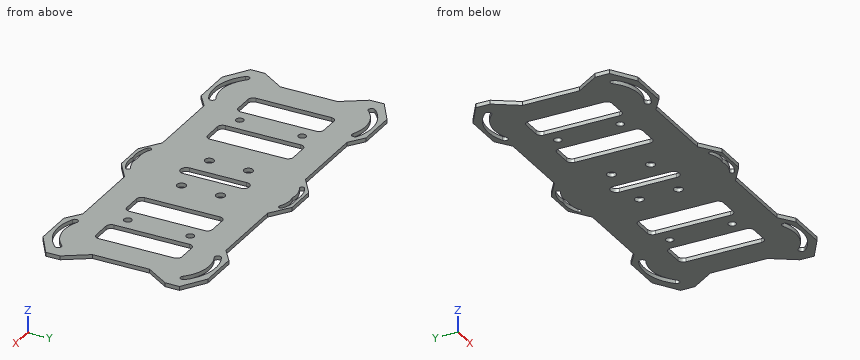
```python
from build123d import *

# Parameters (mm, degrees)
SCHIZZO1_R                   = 1.5
ESTRUSIONE_ESTRUSIONE1_DEPTH = 0.75
SKETCH1_R                    = 1.75
CUT_EXTRUDE1_DEPTH           = 1
CUT_EXTRUDE1_DEPTH_BACK      = 2.5


with BuildPart() as part:
    # Schizzo1 → Estrusione-Estrusione1 (new body, symmetric)
    with BuildSketch(Plane.XY):
        Polygon((-43.5, -27.5), (-13.615232638, -27.5), (-5.964504028, -32.859521299), (5.964504028, -32.859521299), (13.615232638, -27.5), (43.5, -27.5), (49.293787181, -31.722358535), (64.293787181, -31.722358535), (73.508072858, -25.714285677), (73.508072858, -20.214285677), (67.5, -11), (67.5, 11), (73.508072858, 20.214285677), (73.508072858, 25.714285677), (64.293787181, 31.722358535), (49.293787181, 31.722358535), (43.5, 27.5), (13.615232638, 27.5), (5.964504028, 32.859521299), (-5.964504028, 32.859521299), (-13.615232638, 27.5), (-43.5, 27.5), (-49.293787181, 31.722358535), (-64.293787181, 31.722358535), (-73.508072858, 25.714285677), (-73.508072858, 20.214285677), (-67.5, 11), (-67.5, -11), (-73.508072858, -20.214285677), (-73.508072858, -25.714285677), (-64.293787181, -31.722358535), (-49.293787181, -31.722358535), align=None)
        with BuildLine():
            ThreePointArc((-48.754479002, -28.623738791), (-59.172775767, -30.009764998), (-68.405644393, -24.988200197))
            ThreePointArc((-68.405644393, -24.988200197), (-68.356417198, -23.226138607), (-66.594355607, -23.275365801))
            ThreePointArc((-66.594355607, -23.275365801), (-58.719274878, -27.558458065), (-49.83309536, -26.376261209))
            ThreePointArc((-49.83309536, -26.376261209), (-48.17004839, -26.960691821), (-48.754479002, -28.623738791))
        make_face(mode=Mode.SUBTRACT)
        with Locations((-40.191447808, -12)):
            Circle(SCHIZZO1_R, mode=Mode.SUBTRACT)
        with BuildLine():
            ThreePointArc((0, -31.496185519), (-4.133745369, -31.563971562), (-8.018095478, -30.148249145))
            ThreePointArc((-8.018095478, -30.148249145), (-8.326872952, -28.953648185), (-7.132271992, -28.644870711))
            ThreePointArc((-7.132271992, -28.644870711), (-3.764579281, -29.856257566), (-0.187146253, -29.75240554))
            ThreePointArc((-0.187146253, -29.75240554), (0, -29.732097651), (0.187146253, -29.75240554))
            ThreePointArc((0.187146253, -29.75240554), (3.764579281, -29.856257566), (7.132271992, -28.644870711))
            ThreePointArc((7.132271992, -28.644870711), (8.326872952, -28.953648185), (8.018095478, -30.148249145))
            ThreePointArc((8.018095478, -30.148249145), (4.133745369, -31.563971562), (0, -31.496185519))
        make_face(mode=Mode.SUBTRACT)
        with BuildLine():
            ThreePointArc((66.594355607, -23.275365801), (68.356417198, -23.226138607), (68.405644393, -24.988200197))
            ThreePointArc((68.405644393, -24.988200197), (59.172775767, -30.009764998), (48.754479002, -28.623738791))
            ThreePointArc((48.754479002, -28.623738791), (48.17004839, -26.960691821), (49.83309536, -26.376261209))
            ThreePointArc((49.83309536, -26.376261209), (58.719274878, -27.558458065), (66.594355607, -23.275365801))
        make_face(mode=Mode.SUBTRACT)
        with Locations((40.191447808, -12)):
            Circle(SCHIZZO1_R, mode=Mode.SUBTRACT)
        with BuildLine():
            Line((-47.5, -16.5), (-54.5, -16.5))
            ThreePointArc((-54.5, -16.5), (-55.914213562, -15.914213562), (-56.5, -14.5))
            Line((-56.5, -14.5), (-56.5, 14.5))
            ThreePointArc((-56.5, 14.5), (-55.914213562, 15.914213562), (-54.5, 16.5))
            Line((-54.5, 16.5), (-47.5, 16.5))
            ThreePointArc((-47.5, 16.5), (-46.085786438, 15.914213562), (-45.5, 14.5))
            Line((-45.5, 14.5), (-45.5, -14.5))
            ThreePointArc((-45.5, -14.5), (-46.085786438, -15.914213562), (-47.5, -16.5))
        make_face(mode=Mode.SUBTRACT)
        with Locations((-40.191447808, 12)):
            Circle(SCHIZZO1_R, mode=Mode.SUBTRACT)
        with BuildLine():
            Line((-25.5, -16.5), (-32.5, -16.5))
            ThreePointArc((-32.5, -16.5), (-33.914213562, -15.914213562), (-34.5, -14.5))
            Line((-34.5, -14.5), (-34.5, 14.5))
            ThreePointArc((-34.5, 14.5), (-33.914213562, 15.914213562), (-32.5, 16.5))
            Line((-32.5, 16.5), (-25.5, 16.5))
            ThreePointArc((-25.5, 16.5), (-24.085786438, 15.914213562), (-23.5, 14.5))
            Line((-23.5, 14.5), (-23.5, -14.5))
            ThreePointArc((-23.5, -14.5), (-24.085786438, -15.914213562), (-25.5, -16.5))
        make_face(mode=Mode.SUBTRACT)
        with BuildLine():
            ThreePointArc((-2.261398956, 11), (0, 13.261398956), (2.261398956, 11))
            Line((2.261398956, 11), (2.261398956, -11))
            ThreePointArc((2.261398956, -11), (0, -13.261398956), (-2.261398956, -11))
            Line((-2.261398956, -11), (-2.261398956, 11))
        make_face(mode=Mode.SUBTRACT)
        with BuildLine():
            ThreePointArc((-66.594355607, 23.275365801), (-68.356417198, 23.226138607), (-68.405644393, 24.988200197))
            ThreePointArc((-68.405644393, 24.988200197), (-67.961138694, 25.440973547), (-67.5, 25.876794757))
            ThreePointArc((-67.5, 25.876794757), (-58.546813094, 30.113494239), (-48.754479002, 28.623738791))
            ThreePointArc((-48.754479002, 28.623738791), (-48.17004839, 26.960691821), (-49.83309536, 26.376261209))
            ThreePointArc((-49.83309536, 26.376261209), (-58.719274878, 27.558458065), (-66.594355607, 23.275365801))
        make_face(mode=Mode.SUBTRACT)
        with BuildLine():
            ThreePointArc((25.5, -16.5), (24.085786438, -15.914213562), (23.5, -14.5))
            Line((23.5, -14.5), (23.5, 14.5))
            ThreePointArc((23.5, 14.5), (24.085786438, 15.914213562), (25.5, 16.5))
            Line((25.5, 16.5), (32.5, 16.5))
            ThreePointArc((32.5, 16.5), (33.914213562, 15.914213562), (34.5, 14.5))
            Line((34.5, 14.5), (34.5, -14.5))
            ThreePointArc((34.5, -14.5), (33.914213562, -15.914213562), (32.5, -16.5))
            Line((32.5, -16.5), (25.5, -16.5))
        make_face(mode=Mode.SUBTRACT)
        with BuildLine():
            ThreePointArc((47.5, -16.5), (46.085786438, -15.914213562), (45.5, -14.5))
            Line((45.5, -14.5), (45.5, 14.5))
            ThreePointArc((45.5, 14.5), (46.085786438, 15.914213562), (47.5, 16.5))
            Line((47.5, 16.5), (54.5, 16.5))
            ThreePointArc((54.5, 16.5), (55.914213562, 15.914213562), (56.5, 14.5))
            Line((56.5, 14.5), (56.5, -14.5))
            ThreePointArc((56.5, -14.5), (55.914213562, -15.914213562), (54.5, -16.5))
            Line((54.5, -16.5), (47.5, -16.5))
        make_face(mode=Mode.SUBTRACT)
        with Locations((40.191447808, 12)):
            Circle(SCHIZZO1_R, mode=Mode.SUBTRACT)
        with BuildLine():
            ThreePointArc((0.187146253, 29.75240554), (0, 29.732097651), (-0.187146253, 29.75240554))
            ThreePointArc((-0.187146253, 29.75240554), (-3.764579281, 29.856257566), (-7.132271992, 28.644870711))
            ThreePointArc((-7.132271992, 28.644870711), (-8.326872952, 28.953648185), (-8.018095478, 30.148249145))
            ThreePointArc((-8.018095478, 30.148249145), (-4.133745369, 31.563971562), (0, 31.496185519))
            ThreePointArc((0, 31.496185519), (4.133745369, 31.563971562), (8.018095478, 30.148249145))
            ThreePointArc((8.018095478, 30.148249145), (8.326872952, 28.953648185), (7.132271992, 28.644870711))
            ThreePointArc((7.132271992, 28.644870711), (3.764579281, 29.856257566), (0.187146253, 29.75240554))
        make_face(mode=Mode.SUBTRACT)
        with BuildLine():
            ThreePointArc((48.754479002, 28.623738791), (59.172775767, 30.009764998), (68.405644393, 24.988200197))
            ThreePointArc((68.405644393, 24.988200197), (68.356417198, 23.226138607), (66.594355607, 23.275365801))
            ThreePointArc((66.594355607, 23.275365801), (58.719274878, 27.558458065), (49.83309536, 26.376261209))
            ThreePointArc((49.83309536, 26.376261209), (48.17004839, 26.960691821), (48.754479002, 28.623738791))
        make_face(mode=Mode.SUBTRACT)
    extrude(amount=ESTRUSIONE_ESTRUSIONE1_DEPTH, both=True)

    # Sketch1 → Cut-Extrude1 (cut, two sides)
    with BuildSketch(Plane(origin=(0, 0, -0.75), x_dir=(-1, 0, 0), z_dir=(0, 0, -1))) as cut_extrude1_sk:
        with Locations((-10, 7.5)):
            Circle(SKETCH1_R)
        with Locations((-10, -7.5)):
            Circle(SKETCH1_R)
        with Locations((10, -7.5)):
            Circle(SKETCH1_R)
        with Locations((10, 7.5)):
            Circle(SKETCH1_R)
    extrude(amount=CUT_EXTRUDE1_DEPTH, mode=Mode.SUBTRACT)
    extrude(cut_extrude1_sk.sketch, amount=-CUT_EXTRUDE1_DEPTH_BACK, mode=Mode.SUBTRACT)


solid = part.part
```
For this review, take the finished solid that the model builds, in its own axes (mm). Give positions to 0.01 mm unless a question says otherwise; leave off trailing zeros. Write each loop counter-clockwise with the first axis right and the second up, starting at its lowest first coordinate (ties: lowest second). Pieces come first, ordered by that corner, then holes.
Item 1: Take a section at B-B (x = -52.5). Give the boundary of the cut face in (y, z).
Item 2: Take a section at C-C (x = -10). Give the boundary of the cut face in (y, z), and give its area (3 significant figures).
Item 3: Take a section at D-D (z = -0.25). Give the number of separate pieces and of enclosed holes in the cut face, and give its area (3 significant figures).
Item 4: Insertion check: P1, Ø0.8, axis at x = -60.5, z = -0.5, coming from the +Y side; P2, Ø0.8, axis at x = 32.5, z = -0.5, coming from the +Y side. Each pin has a flat end and moves straight along its axis. Give the tip position at first contact, or say it passes through.
Item 5: Wall thickness on probe 1 along X at (y, z) = (0, 0.65); probe 2 along Y at (x, z) = (32.5, 0.65); probe 3 along Y at (x, z) = (-50, -0.35): over which ranges is each line inside the solid? List them lowest first.
Item 6: Take a section at A-A (x = -29.5). Give the boundary of the cut face in (y, z).
Established:
1. outline: (-31.72, -0.75) - (-29.91, -0.75) - (-29.91, 0.75) - (-31.72, 0.75) - close; (-27.35, -0.75) - (-16.5, -0.75) - (-16.5, 0.75) - (-27.35, 0.75) - close; (16.5, -0.75) - (27.35, -0.75) - (27.35, 0.75) - (16.5, 0.75) - close; (29.91, -0.75) - (31.72, -0.75) - (31.72, 0.75) - (29.91, 0.75) - close
2. outline: (-30.03, -0.75) - (-9.25, -0.75) - (-9.25, 0.75) - (-30.03, 0.75) - close; (-5.75, -0.75) - (5.75, -0.75) - (5.75, 0.75) - (-5.75, 0.75) - close; (9.25, -0.75) - (30.03, -0.75) - (30.03, 0.75) - (9.25, 0.75) - close
2. area: 79.6 mm2
3. separate pieces: 1
3. enclosed holes: 19
3. area: 6,370 mm2
4. P1: stops at y = 31.72
4. P2: stops at y = 27.5
5. probe 1: x = -67.5 to -56.5, -45.5 to -34.5, -23.5 to -2.26, 2.26 to 23.5, 34.5 to 45.5, 56.5 to 67.5
5. probe 2: y = -27.5 to -16.5, 16.5 to 27.5
5. probe 3: y = -31.72 to -29.16, -26.46 to -16.5, 16.5 to 26.46, 29.16 to 31.72
6. outline: (-27.5, -0.75) - (-16.5, -0.75) - (-16.5, 0.75) - (-27.5, 0.75) - close; (16.5, -0.75) - (27.5, -0.75) - (27.5, 0.75) - (16.5, 0.75) - close
